from build123d import *

# Parameters (mm, degrees)
SKETCH1_R           = 2.5
BOSS_EXTRUDE1_DEPTH = 4.8
BOSS_EXTRUDE2_DEPTH = 101
SKETCH4_R           = 19.05
BOSS_EXTRUDE3_DEPTH = 1.8
SKETCH5_R           = 4
BOSS_EXTRUDE4_DEPTH = 20.2
CUT_EXTRUDE1_DEPTH  = 15.5
SKETCH8_R           = 28
BOSS_EXTRUDE5_DEPTH = 3
SKETCH9_R           = 2.5
BOSS_EXTRUDE6_DEPTH = 8.2
SKETCH10_R          = 28
BOSS_EXTRUDE7_DEPTH = 20.8
SKETCH11_W          = 21
SKETCH11_H          = 9
BOSS_EXTRUDE8_DEPTH = 17
CHAMFER1_SIZE       = 1
SKETCH12_R          = 4
BOSS_EXTRUDE9_DEPTH = 29


with BuildPart() as part:
    # Sketch1 → Boss-Extrude1 (new body)
    with BuildSketch(Plane.XY):
        with BuildLine():
            Line((-27, -30), (27, -30))
            ThreePointArc((27, -30), (29.121320344, -29.121320344), (30, -27))
            Line((30, -27), (30, 27))
            ThreePointArc((30, 27), (29.121320344, 29.121320344), (27, 30))
            Line((27, 30), (-27, 30))
            ThreePointArc((-27, 30), (-29.121320344, 29.121320344), (-30, 27))
            Line((-30, 27), (-30, -27))
            ThreePointArc((-30, -27), (-29.121320344, -29.121320344), (-27, -30))
        make_face()
        with Locations((-23.57, 23.57)):
            Circle(SKETCH1_R, mode=Mode.SUBTRACT)
        with Locations((23.57, 23.57)):
            Circle(SKETCH1_R, mode=Mode.SUBTRACT)
        with Locations((23.57, -23.57)):
            Circle(SKETCH1_R, mode=Mode.SUBTRACT)
        with Locations((-23.57, -23.57)):
            Circle(SKETCH1_R, mode=Mode.SUBTRACT)
    extrude(amount=-BOSS_EXTRUDE1_DEPTH)

    # Sketch3 → Boss-Extrude2 (add)
    with BuildSketch(Plane(origin=(0, 0, -4.8), x_dir=(-1, 0, 0), z_dir=(0, 0, -1))):
        with BuildLine():
            Line((18, 30), (-18, 30))
            ThreePointArc((-18, 30), (-19.414213562, 29.414213562), (-20, 28))
            Line((-20, 28), (-20, 22))
            ThreePointArc((-20, 22), (-20.585786438, 20.585786438), (-22, 20))
            Line((-22, 20), (-28, 20))
            ThreePointArc((-28, 20), (-29.414213562, 19.414213562), (-30, 18))
            Line((-30, 18), (-30, -18))
            ThreePointArc((-30, -18), (-29.414213562, -19.414213562), (-28, -20))
            Line((-28, -20), (-22, -20))
            ThreePointArc((-22, -20), (-20.585786438, -20.585786438), (-20, -22))
            Line((-20, -22), (-20, -28))
            ThreePointArc((-20, -28), (-19.414213562, -29.414213562), (-18, -30))
            Line((-18, -30), (18, -30))
            ThreePointArc((18, -30), (19.414213562, -29.414213562), (20, -28))
            Line((20, -28), (20, -22))
            ThreePointArc((20, -22), (20.585786438, -20.585786438), (22, -20))
            Line((22, -20), (28, -20))
            ThreePointArc((28, -20), (29.414213562, -19.414213562), (30, -18))
            Line((30, -18), (30, 18))
            ThreePointArc((30, 18), (29.414213562, 19.414213562), (28, 20))
            Line((28, 20), (22, 20))
            ThreePointArc((22, 20), (20.585786438, 20.585786438), (20, 22))
            Line((20, 22), (20, 28))
            ThreePointArc((20, 28), (19.414213562, 29.414213562), (18, 30))
        make_face()
    extrude(amount=BOSS_EXTRUDE2_DEPTH)

    # Sketch4 → Boss-Extrude3 (add)
    with BuildSketch(Plane.XY):
        Circle(SKETCH4_R)
    extrude(amount=BOSS_EXTRUDE3_DEPTH)

    # Sketch5 → Boss-Extrude4 (add)
    with BuildSketch(Plane.XY.offset(1.8)):
        Circle(SKETCH5_R)
    extrude(amount=BOSS_EXTRUDE4_DEPTH)

    # Sketch7 → Cut-Extrude1 (cut)
    with BuildSketch(Plane.XY.offset(22)):
        with BuildLine():
            Line((-1.743559577, 3.6), (1.743559577, 3.6))
            ThreePointArc((1.743559577, 3.6), (0, 4), (-1.743559577, 3.6))
        make_face()
        with BuildLine():
            Line((-3.6, 1.743559577), (-3.6, -1.743559577))
            ThreePointArc((-3.6, -1.743559577), (-4, 0), (-3.6, 1.743559577))
        make_face()
    extrude(amount=-CUT_EXTRUDE1_DEPTH, mode=Mode.SUBTRACT)

    # Sketch8 → Boss-Extrude5 (add)
    with BuildSketch(Plane(origin=(0, 0, -105.8), x_dir=(-1, 0, 0), z_dir=(0, 0, -1))):
        Circle(SKETCH8_R)
    extrude(amount=BOSS_EXTRUDE5_DEPTH)

    # Sketch9 → Boss-Extrude6 (add)
    with BuildSketch(Plane(origin=(0, 0, -108.8), x_dir=(-1, 0, 0), z_dir=(0, 0, -1))):
        with Locations((0, 24)):
            Circle(SKETCH9_R)
        with Locations((20.784609691, 12)):
            Circle(SKETCH9_R)
        with Locations((20.784609691, -12)):
            Circle(SKETCH9_R)
        with Locations((0, -24)):
            Circle(SKETCH9_R)
        with Locations((-20.784609691, -12)):
            Circle(SKETCH9_R)
        with Locations((-20.784609691, 12)):
            Circle(SKETCH9_R)
    extrude(amount=BOSS_EXTRUDE6_DEPTH)

    # Sketch10 → Boss-Extrude7 (add)
    with BuildSketch(Plane(origin=(0, 0, -117), x_dir=(-1, 0, 0), z_dir=(0, 0, -1))):
        Circle(SKETCH10_R)
    extrude(amount=BOSS_EXTRUDE7_DEPTH)

    # Sketch11 → Boss-Extrude8 (add)
    with BuildSketch(Plane(origin=(0, 0, -105.8), x_dir=(-1, 0, 0), z_dir=(0, 0, -1))):
        with Locations((0, -34.5)):
            Rectangle(SKETCH11_W, SKETCH11_H)
    extrude(amount=-BOSS_EXTRUDE8_DEPTH)

    # Chamfer1
    chamfer1_edges = [part.edges().sort_by_distance(p)[0] for p in [
        (10.5, -39, -97.3),
        (-10.5, -39, -97.3),
    ]]
    chamfer(chamfer1_edges, length=CHAMFER1_SIZE)

    # Sketch12 → Boss-Extrude9 (add)
    with BuildSketch(Plane(origin=(0, 0, -137.8), x_dir=(-1, 0, 0), z_dir=(0, 0, -1))):
        Circle(SKETCH12_R)
    extrude(amount=-BOSS_EXTRUDE9_DEPTH)


solid = part.part
CAD build for the part. Positions are in the model's coordinates, mm. A direction names the side the tool comes from. Coordinates: 2 decimals unless noted, no trailing zeros. Write each loop counter-clockwise with the first axis right and the second up, starting at its lowest first coordinate (ties: lowest second). Pieces come first, ordered by that corner, then holes. Notation, with made-up numbers: M 73.5,76.5 L 108.5,76.5 A17 ccw 108.5,92.5 Z; hole C 38.25,-37 d10. An arc over 180 degrees is marked long. Return JSON: item names as keys, results as strings.
Item 1: Two-plate mould, pull along Z, no slides. Class faces 5 (the cylindrical face through (18.475, -12.958, -112.843)), 6 (the flat face through (0, -34, -88.8)), 7 (the cylindrical face through (-25.865, -10.724, -127.254)): +Z half, -Z half, draft (parallel to the pull), parting line (faces both ways), or undercut.
Findings below:
{"face 5": "undercut", "face 6": "+Z half", "face 7": "draft"}
Item 2: Slice it at A-A, the plane z = -55. Write the cut outline in (x, y), and give its area (3 significant figures).
Findings below:
{"outline": "M -30,-18 A2 ccw -28,-20 L -22,-20 A2 cw -20,-22 L -20,-28 A2 ccw -18,-30 L 18,-30 A2 ccw 20,-28 L 20,-22 A2 cw 22,-20 L 28,-20 A2 ccw 30,-18 L 30,18 A2 ccw 28,20 L 22,20 A2 cw 20,22 L 20,28 A2 ccw 18,30 L -18,30 A2 ccw -20,28 L -20,22 A2 cw -22,20 L -28,20 A2 ccw -30,18 Z", "area": "3,200 mm2"}
Item 3: Which spindle directions (+Z, -Z, +X, -X, +Y, -Y) get a long thin tool onto all of the face, cutting with end or side? Do faces 1 (the flat face through (-25, -27, -4.8)), 2 (the flat face through (27, 25, -4.8)), 3 (the cylindrical face through (-15.12, -11.59, 0.89)), 4 (the flat face through (10.5, -34, -97)). Say none if no direction does.
Findings below:
{"face 1": "-Z, -X, -Y", "face 2": "-Z, +X, +Y", "face 3": "+Z", "face 4": "+Z, -Z, +X, -Y"}
Item 4: Slice it at B-B, the plane y = -6. Write the cut outline in (x, z).
Findings below:
{"outline": "M -30,-105.8 L -27.35,-105.8 L -27.35,-108.8 L 27.35,-108.8 L 27.35,-105.8 L 30,-105.8 L 30,0 L 18.08,0 L 18.08,1.8 L -18.08,1.8 L -18.08,0 L -30,0 Z; M -27.35,-137.8 L 27.35,-137.8 L 27.35,-117 L -27.35,-117 Z"}
Item 5: Drop flat-ended pins along their axis: pin 1 Ø16 at (x, z) = (-7, -47) entering from -Y; pin 2 Ø5 at (y, z) = (-26.5, -65) entering from -X; pin 3 Ø7 at (x, y) = (-1.5, -34) entering from +Z. Give the stop position or say it passes through.
Findings below:
{"pin 1": "stops at y = -30", "pin 2": "stops at x = -20", "pin 3": "stops at z = -88.8"}
Item 6: Probe line 1 (Y direction, x = 23.57, z = -1.75); line 2 (Z direction, x = -24, y = -5); line 3 (X direction, y = 23, z = -3). List the from-to ranges inside material, lowest first. Write a range as from..to.
Findings below:
{"line 1": "y = -30..-26.07, -21.07..21.07, 26.07..30", "line 2": "z = -137.8..-117, -108.8..0", "line 3": "x = -30..-26, -21.14..21.14, 26..30"}
